from build123d import *

# Parameters (mm, degrees)
SKETCH_1_R          = 10.4
EXTRUDE_1_DEPTH     = 1.8
SKETCH_2_R          = 11.25
EXTRUDE_2_DEPTH     = 3
SKETCH_3_R          = 3.5
SKETCH_3_R_2        = 2.55
EXTRUDE_3_DEPTH     = 15
SKETCH_3_4_R        = 1.5
CUT_EXTRUDE_2_DEPTH = 4.8
REVOLVE_3_ANGLE     = 30
REVOLVE_4_ANGLE     = 30
EXTRUDE_4_DEPTH     = 2
SKETCH_14_W         = 11.25
SKETCH_14_H         = 3.8


with BuildPart() as part:
    # 草图1 → 凸台-拉伸1 (new body)
    with BuildSketch(Plane(origin=(0, 0, 0), x_dir=(1, 0, 0), z_dir=(0, 1, 0))):
        with Locations(Location((0, 0, 0), (0, 0, 270))):
            Circle(SKETCH_1_R)
    extrude(amount=EXTRUDE_1_DEPTH)

    # 草图2 → 凸台-拉伸2 (add)
    with BuildSketch(Plane(origin=(0, 1.8, 0), x_dir=(1, 0, 0), z_dir=(0, 1, 0))):
        with Locations(Location((0, 0, 0), (0, 0, 270))):
            Circle(SKETCH_2_R)
    extrude(amount=EXTRUDE_2_DEPTH)

    # 草图3 → 凸台-拉伸3 (add)
    with BuildSketch(Plane(origin=(0, 4.8, 0), x_dir=(1, 0, 0), z_dir=(0, 1, 0))):
        with Locations(Location((0, 0, 0), (0, 0, 270))):
            Circle(SKETCH_3_R)
        with Locations(Location((0, 0, 0), (0, 0, 270))):
            Circle(SKETCH_3_R_2, mode=Mode.SUBTRACT)
    extrude(amount=EXTRUDE_3_DEPTH)

    # 草图3<4> → 切除-拉伸2 (cut)
    with BuildSketch(Plane(origin=(0, 4.8, 0), x_dir=(1, 0, 0), z_dir=(0, 1, 0))):
        with Locations(Location((0, 0, 0), (0, 0, 270))):
            Circle(SKETCH_3_4_R)
    extrude(amount=-CUT_EXTRUDE_2_DEPTH, mode=Mode.SUBTRACT)

    # 草图6 → 旋转3 (revolve)
    with BuildSketch(Plane(origin=(0, 0, 0), x_dir=(0, 0, -1), z_dir=(1, 0, 0))):
        Polygon((3.5, 4.8), (3.5, 16.8), (8.5, 4.8), align=None)
        Polygon((-8.5, 4.8), (-3.5, 4.8), (-3.5, 16.8), align=None)
    revolve(axis=Axis((0, 0, 0), (0, 1, 0)), revolution_arc=REVOLVE_3_ANGLE)

    # 草图9 → 旋转4 (revolve)
    with BuildSketch(Plane.XY):
        Polygon((3.5, 4.8), (8.5, 4.8), (3.5, 16.8), align=None)
        Polygon((-8.5, 4.8), (-3.5, 16.8), (-3.5, 4.8), align=None)
    revolve(axis=Axis((0, 0, 0), (0, 1, 0)), revolution_arc=REVOLVE_4_ANGLE)

    # 草图10 → 凸台-拉伸4 (add)
    with BuildSketch(Plane.XZ):
        with BuildLine():
            Line((9.961946981, -0.871557427), (10.858522209, -0.949997596))
            ThreePointArc((10.858522209, -0.949997596), (10.9, 0), (10.858522209, 0.949997596))
            Line((10.858522209, 0.949997596), (9.961946981, 0.871557427))
            ThreePointArc((9.961946981, 0.871557427), (9.84807753, 1.736481777), (9.659258263, 2.588190451))
            Line((9.659258263, 2.588190451), (8.693332437, 2.329371406))
            ThreePointArc((8.693332437, 2.329371406), (9, 0), (8.693332437, -2.329371406))
            Line((8.693332437, -2.329371406), (9.659258263, -2.588190451))
            ThreePointArc((9.659258263, -2.588190451), (9.84807753, -1.736481777), (9.961946981, -0.871557427))
        make_face()
        with BuildLine():
            Line((2.329371406, 8.693332437), (2.588190451, 9.659258263))
            ThreePointArc((2.588190451, 9.659258263), (1.736481777, 9.84807753), (0.871557427, 9.961946981))
            Line((0.871557427, 9.961946981), (0.949997596, 10.858522209))
            ThreePointArc((0.949997596, 10.858522209), (0, 10.9), (-0.949997596, 10.858522209))
            Line((-0.949997596, 10.858522209), (-0.871557427, 9.961946981))
            ThreePointArc((-0.871557427, 9.961946981), (-1.736481777, 9.84807753), (-2.588190451, 9.659258263))
            Line((-2.588190451, 9.659258263), (-2.329371406, 8.693332437))
            ThreePointArc((-2.329371406, 8.693332437), (0, 9), (2.329371406, 8.693332437))
        make_face()
        with BuildLine():
            Line((-2.329371406, -8.693332437), (-2.588190451, -9.659258263))
            ThreePointArc((-2.588190451, -9.659258263), (-1.736481777, -9.84807753), (-0.871557427, -9.961946981))
            Line((-0.871557427, -9.961946981), (-0.949997596, -10.858522209))
            ThreePointArc((-0.949997596, -10.858522209), (0, -10.9), (0.949997596, -10.858522209))
            Line((0.949997596, -10.858522209), (0.871557427, -9.961946981))
            ThreePointArc((0.871557427, -9.961946981), (1.736481777, -9.84807753), (2.588190451, -9.659258263))
            Line((2.588190451, -9.659258263), (2.329371406, -8.693332437))
            ThreePointArc((2.329371406, -8.693332437), (0, -9), (-2.329371406, -8.693332437))
        make_face()
        with BuildLine():
            Line((-8.693332437, 2.329371406), (-9.659258263, 2.588190451))
            ThreePointArc((-9.659258263, 2.588190451), (-9.84807753, 1.736481777), (-9.961946981, 0.871557427))
            Line((-9.961946981, 0.871557427), (-10.858522209, 0.949997596))
            ThreePointArc((-10.858522209, 0.949997596), (-10.9, 0), (-10.858522209, -0.949997596))
            Line((-10.858522209, -0.949997596), (-9.961946981, -0.871557427))
            ThreePointArc((-9.961946981, -0.871557427), (-9.84807753, -1.736481777), (-9.659258263, -2.588190451))
            Line((-9.659258263, -2.588190451), (-8.693332437, -2.329371406))
            ThreePointArc((-8.693332437, -2.329371406), (-9, 0), (-8.693332437, 2.329371406))
        make_face()
    extrude(amount=EXTRUDE_4_DEPTH)

    # 草图11 → 切除-旋转2 (revolve, cut)
    with BuildSketch(Plane.XY, mode=Mode.PRIVATE) as cut_revolve_2_sk:
        Polygon((9.961946981, -2), (10.9, -2), (10.9, 0), align=None)
    revolve(cut_revolve_2_sk.sketch.rotate(Axis((0, 0, 0), (0, -1, 0)), 275), axis=Axis((0, 0, 0), (0, -1, 0)), mode=Mode.SUBTRACT)

    # 草图14 → 切除-旋转3 (revolve, cut)
    with BuildSketch(Plane(origin=(0, 0, 0), x_dir=(0, 0, -1), z_dir=(1, 0, 0))):
        with Locations((-5.625, -0.1)):
            Rectangle(SKETCH_14_W, SKETCH_14_H)
    revolve(axis=Axis((0, 1.8, 0), (0, -1, 0)), mode=Mode.SUBTRACT)


solid = part.part
Build history of the part. All positions in model axes, mm. A direction names the side the tool comes from. Coordinates: 2 decimals unless noted, no trailing zeros. Order: outer loops, then holes, each group sorted by start corner. A loop starts at its lowest first (then second) coordinate and runs counter-clockwise, first axis right, second up. Notation, with made-up numbers: (-36, 59.5) - (-16, 59.5) arc R31 ccw to (-16, 95.5) - close; hole circle Ø1 at (-26, 75.5). An arc over 180 degrees is marked (long way). Write each question's results on one line, items separated by ' | '. Start each with the question number.
Item 1: Mould opens along Z. For faces 4 (the face through (-4.31, 3.28, 10.39)), 5 (the face through (0, 8, 5)), 6 (the face through (0.154, 12.195, -3.497)), 7 (the face through (4.204, 8.217, -2.427)) say: released by +Z, released by -Z, zero draft, split by the parting line, or undercut.
Item 2: Flat gauge pins, fed straight in: pin 1 (1.5 mm diameter, centred on x = 5, y = 12.5, fed in from +Z); pin 2 (2 mm diameter, centred on x = 2, y = 10.5, fed in from -Z); pin 3 (2.5 mm diameter, centred on x = 0, z = 0, fed in from -Y); pin 4 (5 mm diameter, centred on x = -1, y = 12, fed in from +Z). Where does each tip first touch, or does it go through?
Item 3: Band-saw the part on A-A on y = 15.5. Write the cut outline in (x, z).
Item 4: Tool access for faces 1 (the face through (-4.204, 8.217, 2.427)), 2 (the face through (-2.46, 8.22, -4.26)), 3 (the face through (3, 4.8, -3)): list every direction of +Z, -Z, +X, -X, +Y, -Y with a clear straight run to the whole face (end or side of a thin tool).
Item 5: Band-saw the part on B-B on y = 6.25. Write the cut outline in (x, z), and give its area (3 significant figures).
Numbers:
1) face 4: split by the parting line | face 5: zero draft | face 6: undercut | face 7: released by -Z
2) pin 1: z = 0 | pin 2: z = -3.35 | pin 3: through | pin 4: z = 6.45
3) outline: (-4.04, 0) - (-3.5, 0) arc R3.5 ccw to (-1.75, -3.03) - (-2.02, -3.5) arc R4.04 ccw to (0, -4.04) - (0, -3.5) arc R3.5 ccw to (3.03, -1.75) - (3.5, -2.02) arc R4.04 ccw to (4.04, 0) - (3.5, 0) arc R3.5 ccw to (1.75, 3.03) - (2.02, 3.5) arc R4.04 ccw to (0, 4.04) - (0, 3.5) arc R3.5 ccw to (-3.03, 1.75) - (-3.5, 2.02) arc R4.04 ccw to start; hole circle Ø5.1 at (0, 0)
4) face 1: +Z, +Y | face 2: -X, +Y | face 3: +Y
5) outline: (-7.9, 0) - (-3.5, 0) arc R3.5 ccw to (-1.75, -3.03) - (-3.95, -6.84) arc R7.9 ccw to (0, -7.9) - (0, -3.5) arc R3.5 ccw to (3.03, -1.75) - (6.84, -3.95) arc R7.9 ccw to (7.9, 0) - (3.5, 0) arc R3.5 ccw to (1.75, 3.03) - (3.95, 6.84) arc R7.9 ccw to (0, 7.9) - (0, 3.5) arc R3.5 ccw to (-3.03, 1.75) - (-6.84, 3.95) arc R7.9 ccw to start; hole circle Ø5.1 at (0, 0) | area: 70.5 mm^2
